The listing builds one solid part. Answer for the finished solid, in the listing's coordinates (mm). A direction names the side the tool comes from. Round coordinates to 2 decimals unless told otherwise and drop trailing zeros. Write each loop counter-clockwise with the first axis right and the second up, starting at its lowest first coordinate (ties: lowest second). Pieces come first, ordered by that corner, then holes.
(1) The mould has two halves that part along X. Classify faces 3 (the face through (-5, -40, -2)), 4 (the face through (-10, -20, 0)), 5 (the face through (0.29, -2.46, 2.23)): +X half, -X half, draft (parallel to the pull), parting line (faces both ways), or undercut.
(2) A cutting plane is placed at B-B, the plane y = -31. Give the vertices of the cut face in (x, z), and give its area (3 significant figures).
(3) A cutting plane is placed at A-A, the plane z = 0. Give the vertices of the cut face in (x, y).
(4) Each of these flat-tipped pins is pushed along its axis until it touches: pin 1 Ø3 at (x, y) = (7.5, -15) entering from -Z; pin 2 Ø1.5 at (y, z) = (-22, -2) entering from +X; pin 3 Ø1 at (x, y) = (-5.5, -4.5) entering from -Z; pin 4 Ø10 at (y, z) = (-27, 0) entering from +X. Where does it stop, or does it pass through?
(5) For faces 1 (the face through (-0.1, 0, 2.4)), 2 (the face through (4.77, -35.91, 1.5)), determine the directions among +Z, -Z, +X, -X, +Y, -Y from which every point of the face is accessible in a straight line to the end or side of a thin tool.
(6) Find the intervals of material crossed by probe 1 along Z at (x, y) = (0, -3.8); probe 2 along X at (y, z) = (-17.25, 0), in increasing order.
(7) A cutting plane is placed at C-C, the plane x = -5.75. Give the vertices of the cut face in (y, z).
(8) A cutting plane is placed at D-D, the plane y = -7. Give the vertices of the cut face in (x, z), and give its area (3 significant figures).
from build123d import *

# Parameters (mm, degrees)
F0_R          = 10
F1_DEPTH      = 40
F2_R          = 2.25
F3_DEPTH      = 40
F4_R          = 5
F5_DEPTH      = 35
F6_R          = 5.5
F7_DEPTH      = 10.001
F7_DEPTH_BACK = 10.001


with BuildPart() as f1:
    # F0 (on Front) → F1 (new body)
    with BuildSketch(Plane.XZ):
        Circle(F0_R)
    extrude(amount=F1_DEPTH)

    # F2 (on face) → F3 (cut, through all)
    with BuildSketch(Plane(origin=(0, 0, 0), x_dir=(-1, 0, 0), z_dir=(0, 1, 0))):
        Circle(F2_R)
    extrude(amount=-F3_DEPTH, mode=Mode.SUBTRACT)

    # F4 (on face) → F5 (cut)
    with BuildSketch(Plane.XZ.offset(40)):
        Circle(F4_R)
    extrude(amount=-F5_DEPTH, mode=Mode.SUBTRACT)

    # F6 (on Right) → F7 (cut, two sides)
    with BuildSketch(Plane.YZ) as f7_sk:
        with Locations((-27, 0)):
            Circle(F6_R)
    extrude(amount=-F7_DEPTH, mode=Mode.SUBTRACT)
    extrude(f7_sk.sketch, amount=F7_DEPTH_BACK, mode=Mode.SUBTRACT)


solid = f1.part
Solutions:
1. face 3: draft
1. face 4: parting line
1. face 5: undercut
2. outline: (-9.26, -3.77) arc R10 ccw to (9.26, -3.77) - (3.28, -3.77) arc R5 cw to (-3.28, -3.77) - close; (-9.26, 3.77) - (-3.28, 3.77) arc R5 cw to (3.28, 3.77) - (9.26, 3.77) arc R10 ccw to start
2. area: 156 mm2
3. outline: (-10, -40) - (-5, -40) - (-5, -32.5) - (-10, -32.5) - close; (-10, -21.5) - (-5, -21.5) - (-5, -5) - (-2.25, -5) - (-2.25, 0) - (-10, 0) - close; (2.25, -5) - (5, -5) - (5, -21.5) - (10, -21.5) - (10, 0) - (2.25, 0) - close; (5, -40) - (10, -40) - (10, -32.5) - (5, -32.5) - close
4. pin 1: stops at z = -8
4. pin 2: stops at x = 9.91
4. pin 3: stops at z = -8.66
4. pin 4: passes through
5. face 1: +Z, -Z, +X, -X, +Y
5. face 2: -Y
6. probe 1: z = -10 to -2.25, 2.25 to 10
6. probe 2: x = -10 to -5, 5 to 10
7. outline: (-40, -8.18) - (0, -8.18) - (0, 8.18) - (-40, 8.18) - close; hole circle Ø11 at (-27, 0)
8. outline: circle Ø20 at (0, 0); hole circle Ø10 at (0, 0)
8. area: 236 mm2
